```python
from build123d import *

# Parameters (mm, degrees)
F0_R           = 31.75
F1_DEPTH       = 2.54
F2_R           = 19.05
F3_DEPTH       = 20.32
F4_R           = 31.75
F4_R_2         = 19.05
F5_DEPTH       = 2.54
F6_R           = 9.525
F7_DEPTH       = 2.54
F8_R           = 9.525
F9_DEPTH       = 2.54
F10_R          = 3.429
F11_DEPTH      = 30.48
F12_R          = 0.9525
F13_DEPTH      = 25.4
F13_DEPTH_BACK = 25.4


with BuildPart() as f1:
    # F0 (on Top) → F1 (new body)
    with BuildSketch(Plane.XY):
        Circle(F0_R)
    extrude(amount=F1_DEPTH)

    # F2 (on face) → F3 (join)
    with BuildSketch(Plane.XY.offset(2.54)):
        Circle(F2_R)
    extrude(amount=F3_DEPTH)

    # F4 (on face) → F5 (join)
    with BuildSketch(Plane.XY.offset(22.86)):
        Circle(F4_R)
        Circle(F4_R_2, mode=Mode.SUBTRACT)
        Circle(F4_R_2)
    extrude(amount=F5_DEPTH)

    # F6 (on face) → F7 (join)
    with BuildSketch(Plane.XY.offset(25.4)):
        Circle(F6_R)
    extrude(amount=F7_DEPTH)

    # F8 (on face) → F9 (join)
    with BuildSketch(Plane(origin=(0, 0, 0), x_dir=(1, 0, 0), z_dir=(0, 0, -1))):
        Circle(F8_R)
    extrude(amount=F9_DEPTH)

    # F10 (on face) → F11 (cut)
    with BuildSketch(Plane(origin=(0, 0, -2.54), x_dir=(1, 0, 0), z_dir=(0, 0, -1))):
        Circle(F10_R)
    extrude(amount=-F11_DEPTH, mode=Mode.SUBTRACT)

    # F12 (on Front) → F13 (cut, two sides)
    with BuildSketch(Plane.XZ) as f13_sk:
        with Locations((0, 12.7)):
            Circle(F12_R)
    extrude(amount=-F13_DEPTH, mode=Mode.SUBTRACT)
    extrude(f13_sk.sketch, amount=F13_DEPTH_BACK, mode=Mode.SUBTRACT)


solid = f1.part
```
Part model, mm, in its own coordinate system. A direction names the side the tool comes from. Round coordinates to 2 decimals unless told otherwise and drop trailing zeros. Loops run counter-clockwise (first coordinate to the right, second up) from the corner with the lowest first, then second, coordinate; pieces in that order, holes last. Notation, with made-up numbers: (77.5, 53) -> (134.5, 53) arc R11 ccw to (134.5, 74) -> close; hole circle Ø3 at (19, 49.5). An arc over 180 degrees is marked (long way). Use a Markdown table: item, result.
1) Cut at B-B, the plane x = 0. State how many separate pieces and enclosed holes the cut face has, and give its area (3 significant figures).
The answers:
| item | result |
|---|---|
| separate pieces | 4 |
| enclosed holes | 0 |
| area | 925 mm2 |
2) Pull direction Z, two halves, no side cores. Call faces 1 (the flat face through (4, 0, 27.94)), 2 (the cylindrical face through (-15.12, -11.59, 12.56)), 3 (the cylindrical face through (-6.883, -30.995, 24.112)): pulls with the +Z half, pulls with the -Z half, needs draft (parallel to the pull), parting line crosses it, or undercut.
The answers:
| item | result |
|---|---|
| face 1 | pulls with the +Z half |
| face 2 | undercut |
| face 3 | needs draft |
3) Cut at C-C, the plane x = -27. List the corners of the cut face in (y, z).
The answers:
| item | result |
|---|---|
| outline | (-16.71, 0) -> (16.71, 0) -> (16.71, 2.54) -> (-16.71, 2.54) -> close; (-16.71, 22.86) -> (16.71, 22.86) -> (16.71, 25.4) -> (-16.71, 25.4) -> close |
4) Cut at A-A, the plane y = 0. List the corners of the cut face in (x, z) (3 decimals), and give its area (3 significant figures).
The answers:
| item | result |
|---|---|
| outline | (-31.75, 0) -> (-9.525, 0) -> (-9.525, -2.54) -> (-3.429, -2.54) -> (-3.429, 27.94) -> (-9.525, 27.94) -> (-9.525, 25.4) -> (-31.75, 25.4) -> (-31.75, 22.86) -> (-19.05, 22.86) -> (-19.05, 2.54) -> (-31.75, 2.54) -> close; (3.429, -2.54) -> (9.525, -2.54) -> (9.525, 0) -> (31.75, 0) -> (31.75, 2.54) -> (19.05, 2.54) -> (19.05, 22.86) -> (31.75, 22.86) -> (31.75, 25.4) -> (9.525, 25.4) -> (9.525, 27.94) -> (3.429, 27.94) -> close |
| area | 985 mm2 |
5) Drop flat-ended pins along their axis: pin 1 Ø10 at (x, z) = (14.5, 5) entering from +Y; pin 2 Ø6 at (y, z) = (3, 12) entering from +X; pin 3 Ø6 at (y, z) = (-20, 4) entering from +X. Give the stop position or say it passes through.
The answers:
| item | result |
|---|---|
| pin 1 | stops at y = 30.08 |
| pin 2 | stops at x = 19.05 |
| pin 3 | stops at x = 26.57 |
6) Probe line 1 (Z direction, x = -9, y = 27); line 2 (Z direction, x = 0, y = -12.75); line 3 (Y direction, x = 0, z = 18). List the from-to ranges inside material, lowest first. Write a range as [from, to].
The answers:
| item | result |
|---|---|
| line 1 | z = [0, 2.54], [22.86, 25.4] |
| line 2 | z = [0, 11.75], [13.65, 25.4] |
| line 3 | y = [-19.05, -3.43], [3.43, 19.05] |
7) Tool access for faces 4 (the flat face through (14, -14, 2.54)), 5 (the flat face through (7, 8, 25.4)), 6 (the flat face through (7, 8, 0)): list every direction of +Z, -Z, +X, -X, +Y, -Y with a clear straight run to the whole face (end or side of a thin tool).
The answers:
| item | result |
|---|---|
| face 4 | none |
| face 5 | +Z |
| face 6 | -Z |
